Read the model definition and answer for the solid it produces. Units are mm, in the model's axes. Face numbers are marked on the shaded views. A direction names the side the tool comes from. Coordinates: 2 decimals unless noted, no trailing zeros. Write each loop counter-clockwise with the first axis right and the second up, starting at its lowest first coordinate (ties: lowest second). Pieces come first, ordered by that corner, then holes. Notation, with made-up numbers: (45, 78) -> (87, 78) arc R20 cw to (87, 84) -> close; hole circle Ø7 at (85, 74). An arc over 180 degrees is marked (long way). Answer in a Markdown table with one row per item. Add a question column.
Item 1: Section B-B on y = 2.5 is taken. Count the separate pieces of the cut face and the enclosed holes in it, then the cut area to 3 significant figures.
Item 2: For a pull along X with two mould halves and no side action, classify the marked faces 1, 2 and 3 as +X half, -X half, draft (parallel to the pull), parting line (faces both ways), or undercut.
Item 3: Which of the six approach directions +Z, -Z, +X, -X, +Y, -Y give full straight-line access (tool end or side, diameter ignored) to the marked faces 4 and 5?
Item 4: Section A-A on z = -25 is taken. Write down the section's boundary in (x, y) (3 decimals).
Item 5: Given pin 1 Ø0.8 at (x, z) = (26, -1) entering from +Y (3 decimals); pin 2 Ø4 at (x, z) = (17.5, -58) entering from -Y; pin 3 Ø0.5 at (x, y) = (21, 2) entering from +Z; pin 4 Ø1.6 at (x, z) = (26, -13) entering from +Y (3 decimals), each flat-ended and moving along its own axis, determine where each tip first touches the part or whether it passes through.
Item 6: Section D-D on z = -36.5 is taken. Write down the section's boundary in (x, y) (3 decimals), then the cut area to 3 significant figures.
Item 7: Straight lines are drawn through the part: line 1 (X direction, y = 1.75, z = -21.5) (3 decimals); line 2 (X direction, y = 1.25, z = -25.5); line 3 (X direction, y = 1.5, z = -50). For each, find the intervals that lie inside material, in ascending order. Write a range as from..to.
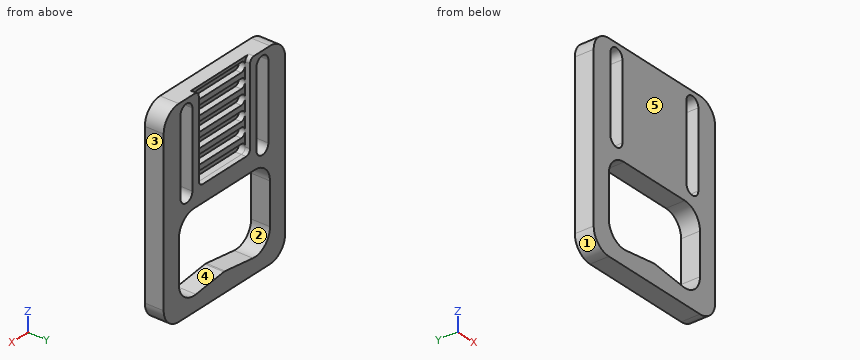
```python
from build123d import *

# Parameters (mm, degrees)
SKETCH1_W           = 50.8
SKETCH1_H           = 66.675
BOSS_EXTRUDE1_DEPTH = 3.175
FILLET1_R           = 6.35
SKETCH3_W           = 21.450000026
SKETCH3_H           = 29.20000002
CUT_EXTRUDE2_DEPTH  = 1.650000002
CUT_EXTRUDE1_DEPTH  = 2.100000118
FILLET2_R           = 1.600000102


with BuildPart() as part:
    # Sketch1 → Boss-Extrude1 (new, symmetric)
    with BuildSketch(Plane(origin=(0, 0, 0), x_dir=(1, 0, 0), z_dir=(0, 1, 0))):
        with Locations((25.4, 33.3375)):
            Rectangle(SKETCH1_W, SKETCH1_H)
        with BuildLine():
            ThreePointArc((7.0358, 29.36875), (9.525, 31.85795), (12.0142, 29.36875))
            Line((12.0142, 29.36875), (12.0142, 3.96875))
            ThreePointArc((12.0142, 3.96875), (9.525, 1.47955), (7.0358, 3.96875))
            Line((7.0358, 3.96875), (7.0358, 29.36875))
        make_face(mode=Mode.SUBTRACT)
        with BuildLine():
            ThreePointArc((38.7858, 29.36875), (41.275, 31.85795), (43.7642, 29.36875))
            Line((43.7642, 29.36875), (43.7642, 3.96875))
            ThreePointArc((43.7642, 3.96875), (41.275, 1.47955), (38.7858, 3.96875))
            Line((38.7858, 3.96875), (38.7858, 29.36875))
        make_face(mode=Mode.SUBTRACT)
        with BuildLine():
            Line((6.35, 34.925), (6.35, 62.45225))
            Line((6.35, 62.45225), (25.151930523, 60.102008685))
            ThreePointArc((25.151930523, 60.102008685), (25.4, 60.086564438), (25.648069477, 60.102008685))
            Line((25.648069477, 60.102008685), (44.45, 62.45225))
            Line((44.45, 62.45225), (44.45, 34.925))
            Line((44.45, 34.925), (6.35, 34.925))
        make_face(mode=Mode.SUBTRACT)
    extrude(amount=BOSS_EXTRUDE1_DEPTH, both=True)

    # Fillet1
    fillet1_edges = [part.edges().sort_by_distance(p)[0] for p in [
        (6.35, 0, -62.45225),
        (6.35, 0, -34.925),
        (44.45, 0, -34.925),
        (44.45, 0, -62.45225),
        (0, 0, 0),
        (0, 0, -66.675),
        (50.8, 0, -66.675),
        (50.8, 0, 0),
    ]]
    fillet(fillet1_edges, radius=FILLET1_R)

    # Sketch3 → Cut-Extrude2 (cut)
    with BuildSketch(Plane(origin=(0, 3.175, 0), x_dir=(1, 0, 0), z_dir=(0, 1, 0))):
        with Locations((25.4, 14.60000001)):
            Rectangle(SKETCH3_W, SKETCH3_H)
    extrude(amount=-CUT_EXTRUDE2_DEPTH, mode=Mode.SUBTRACT)

    # Sketch2 → Cut-Extrude1 (cut)
    with BuildSketch(Plane(origin=(0, 1.524999998, 0), x_dir=(1, 0, 0), z_dir=(0, 1, 0))):
        with BuildLine():
            Line((16.274999962, 4.199999982), (34.525000038, 4.199999982))
            ThreePointArc((34.525000038, 4.199999982), (36.125000013, 2.600000007), (34.525000038, 1.000000032))
            Line((34.525000038, 1.000000032), (16.274999962, 1.000000032))
            ThreePointArc((16.274999962, 1.000000032), (14.674999987, 2.600000007), (16.274999962, 4.199999982))
        make_face()
        with BuildLine():
            Line((16.274999962, 29.199999512), (34.525000038, 29.199999512))
            ThreePointArc((34.525000038, 29.199999512), (36.125000013, 27.599999537), (34.525000038, 25.999999562))
            Line((34.525000038, 25.999999562), (16.274999962, 25.999999562))
            ThreePointArc((16.274999962, 25.999999562), (14.674999987, 27.599999537), (16.274999962, 29.199999512))
        make_face()
        with BuildLine():
            Line((16.274999962, 9.199999888), (34.525000038, 9.199999888))
            ThreePointArc((34.525000038, 9.199999888), (36.125000013, 7.599999913), (34.525000038, 5.999999938))
            Line((34.525000038, 5.999999938), (16.274999962, 5.999999938))
            ThreePointArc((16.274999962, 5.999999938), (14.674999987, 7.599999913), (16.274999962, 9.199999888))
        make_face()
        with BuildLine():
            Line((16.274999962, 14.199999794), (34.525000038, 14.199999794))
            ThreePointArc((34.525000038, 14.199999794), (36.125000013, 12.599999819), (34.525000038, 10.999999844))
            Line((34.525000038, 10.999999844), (16.274999962, 10.999999844))
            ThreePointArc((16.274999962, 10.999999844), (14.674999987, 12.599999819), (16.274999962, 14.199999794))
        make_face()
        with BuildLine():
            Line((16.274999962, 19.1999997), (34.525000038, 19.1999997))
            ThreePointArc((34.525000038, 19.1999997), (36.125000013, 17.599999725), (34.525000038, 15.99999975))
            Line((34.525000038, 15.99999975), (16.274999962, 15.99999975))
            ThreePointArc((16.274999962, 15.99999975), (14.674999987, 17.599999725), (16.274999962, 19.1999997))
        make_face()
        with BuildLine():
            Line((16.274999962, 24.199999606), (34.525000038, 24.199999606))
            ThreePointArc((34.525000038, 24.199999606), (36.125000013, 22.599999631), (34.525000038, 20.999999656))
            Line((34.525000038, 20.999999656), (16.274999962, 20.999999656))
            ThreePointArc((16.274999962, 20.999999656), (14.674999987, 22.599999631), (16.274999962, 24.199999606))
        make_face()
    extrude(amount=-CUT_EXTRUDE1_DEPTH, mode=Mode.SUBTRACT)

    # Fillet2
    fillet2_edges = [part.edges().sort_by_distance(p)[0] for p in [
        (36.125000013, 2.349999999, -29.20000002),
        (14.674999987, 2.349999999, -29.20000002),
    ]]
    fillet(fillet2_edges, radius=FILLET2_R - 0.0001)  # a hair under: the kernel refuses the full size
    fillet2_2_edges = [part.edges().sort_by_distance(p)[0] for p in [
        (36.125000013, 2.349999999, 0),
        (14.674999987, 2.349999999, 0),
    ]]
    fillet(fillet2_2_edges, radius=FILLET2_R)


solid = part.part
```
Results below:
| question | item | result |
|---|---|---|
| 1 | separate pieces | 1 |
| 1 | enclosed holes | 3 |
| 1 | area | 1,470 mm2 |
| 2 | face 1 | -X half |
| 2 | face 2 | undercut |
| 2 | face 3 | +X half |
| 3 | face 4 | +Y, -Y |
| 3 | face 5 | +Z, -Z, +X, -X, -Y |
| 4 | outline | (0, -3.175) -> (7.036, -3.175) -> (7.036, 3.175) -> (0, 3.175) -> close; (12.014, -3.175) -> (38.786, -3.175) -> (38.786, 3.175) -> (36.125, 3.175) -> (36.125, 1.525) -> (14.675, 1.525) -> (14.675, 3.175) -> (12.014, 3.175) -> close; (43.764, -3.175) -> (50.8, -3.175) -> (50.8, 3.175) -> (43.764, 3.175) -> close |
| 5 | pin 1 | stops at y = 1.525 |
| 5 | pin 2 | passes through |
| 5 | pin 3 | stops at z = -29.2 |
| 5 | pin 4 | stops at y = -0.575 |
| 6 | outline | (0, -3.175) -> (8.514, -3.175) -> (8.514, 3.175) -> (0, 3.175) -> close; (42.286, -3.175) -> (50.8, -3.175) -> (50.8, 3.175) -> (42.286, 3.175) -> close |
| 6 | area | 108 mm2 |
| 7 | line 1 | x = 0..7.036, 12.014..14.675, 36.125..38.786, 43.764..50.8 |
| 7 | line 2 | x = 0..7.04, 12.01..38.79, 43.76..50.8 |
| 7 | line 3 | x = 0..6.35, 44.45..50.8 |
